```python
from build123d import *

# Parameters (mm, degrees)
EXTRUSION1_DEPTH             = 8
ESQUISSE2_OUTSIDE_W          = 24.072
ESQUISSE2_OUTSIDE_H          = 29.072
ENL_V_MAT_EXTRU_1_DEPTH      = 4.5
ENL_V_MAT_EXTRU_1_DEPTH_BACK = 12.5
CONG_1_R                     = 0.5
ESQUISSE3_R                  = 2.75
ENL_V_MAT_EXTRU_3_DEPTH      = 22
ESQUISSE4_W                  = 7.923568605
ESQUISSE4_H                  = 0.6
ENL_V_MAT_EXTRU_4_DEPTH      = 22.0000001
ESQUISSE5_R                  = 1.25
ENL_V_MAT_EXTRU_5_DEPTH      = 14
ENL_V_MAT_EXTRU_7_REACH      = 17
ESQUISSE7_R                  = 1.75
ESQUISSE6_R                  = 2.8
ENL_V_MAT_EXTRU_6_DEPTH      = 1


with BuildPart() as part:
    # Esquisse1 → Extrusion1 (new body, symmetric)
    with BuildSketch(Plane(origin=(0, 0, 0), x_dir=(0, 0, -1), z_dir=(1, 0, 0))):
        Polygon((3.5, 0), (-3.5, 0), (-3.5, 21), (11.5, 21), (11.5, 12), align=None)
    extrude(amount=EXTRUSION1_DEPTH, both=True)

    # Esquisse2 outside → Enlèv. mat.-Extru.1 (cut, two sides)
    with BuildSketch(Plane.XY) as enl_v_mat_extru_1_sk:
        with Locations((0, 10.5)):
            Rectangle(ESQUISSE2_OUTSIDE_W, ESQUISSE2_OUTSIDE_H)
        with BuildLine():
            Line((-3.5, 0), (-8, 19))
            ThreePointArc((-8, 19), (0, 21), (8, 19))
            Line((8, 19), (3.5, 0))
            Line((3.5, 0), (-3.5, 0))
        make_face(mode=Mode.SUBTRACT)
    extrude(amount=ENL_V_MAT_EXTRU_1_DEPTH, mode=Mode.SUBTRACT)
    extrude(enl_v_mat_extru_1_sk.sketch, amount=-ENL_V_MAT_EXTRU_1_DEPTH_BACK, mode=Mode.SUBTRACT)

    # Congé1
    cong_1_edges = [part.edges().sort_by_distance(p)[0] for p in [
        (0, 12, -11.5),
        (5.75, 9.5, 3.5),
        (7.171052632, 15.5, -11.5),
        (-7.171052632, 15.5, -11.5),
        (0, 21, -11.5),
        (-8, 19, -4),
        (-5.75, 9.5, 3.5),
        (8, 19, -4),
        (0, 21, 3.5),
        (-4.921052632, 6, -7.5),
        (4.921052632, 6, -7.5),
    ]]
    fillet(cong_1_edges, radius=CONG_1_R)

    # Esquisse3 → Enlèv. mat.-Extru.3 (cut, through all)
    with BuildSketch(Plane(origin=(0, 0, 0), x_dir=(1, 0, 0), z_dir=(0, 1, 0))):
        with Locations(Location((0, 0, 0), (0, 0, 90))):  # turned: the seam where the file's is
            Circle(ESQUISSE3_R)
    extrude(amount=ENL_V_MAT_EXTRU_3_DEPTH, mode=Mode.SUBTRACT)

    # Esquisse4 → Enlèv. mat.-Extru.4 (cut, through all)
    with BuildSketch(Plane(origin=(0, 0, 0), x_dir=(1, 0, 0), z_dir=(0, 1, 0))):
        with Locations((-3.961784303, 0)):
            Rectangle(ESQUISSE4_W, ESQUISSE4_H)
    extrude(amount=ENL_V_MAT_EXTRU_4_DEPTH, mode=Mode.SUBTRACT)

    # Esquisse5 → Enlèv. mat.-Extru.5 (cut)
    with BuildSketch(Plane.XY.offset(3.5)):
        with Locations((-4.2, 14)):
            Circle(ESQUISSE5_R)
    extrude(amount=-ENL_V_MAT_EXTRU_5_DEPTH, mode=Mode.SUBTRACT)

    # Esquisse7 → Enlèv. mat.-Extru.7 (cut, up to next)
    with BuildSketch(Plane.XY.offset(3.5), mode=Mode.PRIVATE) as enl_v_mat_extru_7_sk1:
        with Locations((-4.2, 14)):
            Circle(ESQUISSE7_R)
    enl_v_mat_extru_7_tool1 = extrude(enl_v_mat_extru_7_sk1.sketch, amount=-ENL_V_MAT_EXTRU_7_REACH, mode=Mode.PRIVATE) & part.part
    add(enl_v_mat_extru_7_tool1.solids().sort_by_distance((-4.2, 14, 3.5))[0], mode=Mode.SUBTRACT)

    # Esquisse6 → Enlèv. mat.-Extru.6 (cut)
    with BuildSketch(Plane.XY.offset(3.5)):
        with Locations((-4.2, 14)):
            Circle(ESQUISSE6_R)
    extrude(amount=-ENL_V_MAT_EXTRU_6_DEPTH, mode=Mode.SUBTRACT)


solid = part.part
```
Design review of the part built by this model. Coordinates are the model's own, in mm. A direction names the side the tool comes from. Coordinates: 2 decimals unless noted, no trailing zeros. Loops run counter-clockwise (first coordinate to the right, second up) from the corner with the lowest first, then second, coordinate; pieces in that order, holes last.
Q1. To check wall thickness, follow line 1 (Z direction, x = 0, y = 17.75); line 2 (Z direction, x = 2, y = 19.5); line 3 (X direction, y = 12.5, z = -0.5). State the ranges of each line that lie inside material, in increasing order.
Reported:
line 1: z = -11.5 to -2.75, 2.75 to 3.5
line 2: z = -11.5 to -1.89, 1.89 to 3.5
line 3: x = -6.46 to -2.7, 2.7 to 6.46
Q2. The part is to be moulded in two halves that separate along X. For faces 1 (the face through (-4, 14, -10.5)), 2 (the face through (6.226, 11.51, -2.346)), 3 (the face through (0, 10, 3.5)), 4 (the face through (2.748, 10.353, 0.117)), say which applies: +X half, -X half, draft (parallel to the pull), parting line (faces both ways), or undercut.
Reported:
face 1: undercut
face 2: +X half
face 3: draft
face 4: undercut
Q3. We need section A-A on z = 1.5. State the section outline as (x, y) points, and give its area (3 significant figures).
Reported:
outline: (-7.91, 18.62) - (-3.5, 0) - (-2.3, 0) - (-2.3, 20.84) arc R17 ccw to (-7.65, 19.18) arc R0.5 ccw to start; (2.3, 0) - (3.5, 0) - (7.91, 18.62) arc R0.5 ccw to (7.65, 19.18) arc R17 ccw to (2.3, 20.84) - close; hole circle Ø3.5 at (-4.2, 14)
area: 134 mm2
Q4. For pin 1 (2 mm diameter, centred on x = -4.2, y = 14, fed in from +Z); pin 2 (6 mm diameter, centred on x = -5, y = 5.5, fed in from -Z); pin 3 (8 mm diameter, centred on y = 10, z = 1.5, fed in from +X), all flat-tipped, find the tip position at first contact; note any pin that passes through.
Reported:
pin 1: stops at z = -10.5
pin 2: stops at z = -9.17
pin 3: stops at x = 6.82
Q5. We need section B-B on x = 0. State the section outline as (y, z) points, and give its area (3 significant figures).
Reported:
outline: (0, -3.5) - (11.87, -11.42) arc R0.5 ccw to (12.15, -11.5) - (20.5, -11.5) arc R0.5 ccw to (21, -11) - (21, -2.75) - (0, -2.75) - close; (0, 2.75) - (21, 2.75) - (21, 3) arc R0.5 ccw to (20.5, 3.5) - (0, 3.5) - close
area: 151 mm2
Q6. Tool access review of faces 5 (the face through (-6, 13, 0.3)), 6 (the face through (-1.453, 14.541, 3.007)), 7 (the face through (0, 16, -11.5)): name each direction out of +Z, -Z, +X, -X, +Y, -Y from which nothing blocks a thin tool from reaching the whole face with its end or side.
Reported:
face 5: -X, +Y, -Y
face 6: +Z
face 7: -Z, +X, -X, +Y, -Y
